```python
from build123d import *

# Parameters (mm, degrees)
SKETCH2_W               = 85
SKETCH2_H               = 115
BOSS_EXTRUDE1_DEPTH     = 15
SKETCH3_W               = 15
SKETCH3_H               = 4.5
CUT_EXTRUDE1_DEPTH      = 144.788038445
MIRROR2_COPY_1_SKETCH_W = 15
MIRROR2_COPY_1_SKETCH_H = 4.5
MIRROR2_COPY_1_DEPTH    = 144.788038445
SKETCH4_W               = 55
SKETCH4_H               = 115
BOSS_EXTRUDE2_DEPTH     = 2
SKETCH6_W               = 55
SKETCH6_H               = 115
CUT_EXTRUDE2_DEPTH      = 4.5
SKETCH5_W               = 85
SKETCH5_H               = 115
BOSS_EXTRUDE3_DEPTH     = 4


with BuildPart() as part:
    # Sketch2 → Boss-Extrude1 (new body)
    with BuildSketch(Plane.XY):
        with Locations((42.5, 57.5)):
            Rectangle(SKETCH2_W, SKETCH2_H)
    extrude(amount=BOSS_EXTRUDE1_DEPTH)

    # Sketch3 → Cut-Extrude1 (cut, through all)
    with BuildSketch(Plane(origin=(0, 115, 0), x_dir=(1, 0, 0), z_dir=(0, 1, 0))):
        with Locations((7.5, -12.75)):
            Rectangle(SKETCH3_W, SKETCH3_H)
    cut_extrude1 = extrude(amount=-CUT_EXTRUDE1_DEPTH, mode=Mode.SUBTRACT)

    # Mirror1: Cut-Extrude1 across plane
    add(cut_extrude1.mirror(Plane.XY.offset(7.5)), mode=Mode.SUBTRACT)

    # Mirror2: Cut-Extrude1 across plane
    add(cut_extrude1.mirror(Plane.ZY.offset(-42.5)), mode=Mode.SUBTRACT)

    # Mirror2 copy 1 sketch → Mirror2 copy 1 (cut, through all)
    with BuildSketch(Plane(origin=(85, 115, 15), x_dir=(-1, 0, 0), z_dir=(0, 1, 0))):
        with Locations((7.5, -12.75)):
            Rectangle(MIRROR2_COPY_1_SKETCH_W, MIRROR2_COPY_1_SKETCH_H)
    extrude(amount=-MIRROR2_COPY_1_DEPTH, mode=Mode.SUBTRACT)

    # Sketch4 → Boss-Extrude2 (add)
    with BuildSketch(Plane.XY.offset(15)):
        with Locations((42.5, 57.5)):
            Rectangle(SKETCH4_W, SKETCH4_H)
    extrude(amount=BOSS_EXTRUDE2_DEPTH)

    # Sketch6 → Cut-Extrude2 (cut)
    with BuildSketch(Plane(origin=(0, 0, 0), x_dir=(-1, 0, 0), z_dir=(0, 0, -1))):
        with Locations((-42.5, 57.5)):
            Rectangle(SKETCH6_W, SKETCH6_H)
    extrude(amount=-CUT_EXTRUDE2_DEPTH, mode=Mode.SUBTRACT)

    # Sketch5 → Boss-Extrude3 (add)
    with BuildSketch(Plane.XY.offset(17)):
        with Locations((42.5, 57.5)):
            Rectangle(SKETCH5_W, SKETCH5_H)
    extrude(amount=BOSS_EXTRUDE3_DEPTH)


solid = part.part
```
Input: part model. Units: mm. Frame: model coordinates. A direction names the side the tool comes from. Round coordinates to 2 decimals unless told otherwise and drop trailing zeros. Loops run counter-clockwise (first coordinate to the right, second up) from the corner with the lowest first, then second, coordinate; pieces in that order, holes last. Notation, with made-up numbers: M 88,11.5 L 127,11.5 A10 ccw 127,15.5 Z; hole C 39,8 d8. An arc over 180 degrees is marked long. Answer in a Markdown table with one row per item. Add a question column.
1. Contact query for a flat-ended pin moving along its axis: pin 1 (2 mm diameter, centred on y = 30.5, z = 15, fed in from -X). Output: stop coordinate, or through.
2. Section C-C (z = 15.5). Output: boundary loops of the cut face in (x, y), and give its area (4 significant figures).
3. Section A-A (x = 6). Output: boundary loops of the cut face in (y, z).
4. Set-up query: faces 1 (the face through (15, 57, 14)), 2 (the face through (77, 58, 17)), 3 (the face through (85, 57, 7)). Return all of +Z, -Z, +X, -X, +Y, -Y with unobstructed straight access to the full face (end or side cutting, diameter ignored); none if empty.
5. Section B-B (y = 75). Output: boundary loops of the cut face in (x, z), and give its area (3 significant figures).
6. Mould query, pull axis Z, two halves, no side actions, for faces 4 (the face through (7, 58, 10.5)), 5 (the face through (42, 115, 13)), 6 (the face through (42, 58, 4.5)). Classes: released by +Z, released by -Z, zero draft, split by the parting line, or undercut.
7. Ray query, probe 1 along Z at (x, y) = (7, 26.5); probe 2 along X at (y, z) = (27.5, 16.75). Return the intervals inside material, ascending.
Values follow:
| question | item | result |
|---|---|---|
| 1 | pin 1 | x = 15 |
| 2 | outline | M 15,0 L 70,0 L 70,115 L 15,115 Z |
| 2 | area | 6,325 mm^2 |
| 3 | outline | M 0,4.5 L 115,4.5 L 115,10.5 L 0,10.5 Z; M 0,17 L 115,17 L 115,21 L 0,21 Z |
| 4 | face 1 | -X, +Y, -Y |
| 4 | face 2 | +X, +Y, -Y |
| 4 | face 3 | +Z, -Z, +X, +Y, -Y |
| 5 | outline | M 0,4.5 L 85,4.5 L 85,10.5 L 70,10.5 L 70,17 L 85,17 L 85,21 L 0,21 L 0,17 L 15,17 L 15,10.5 L 0,10.5 Z |
| 5 | area | 1,210 mm^2 |
| 6 | face 4 | undercut |
| 6 | face 5 | zero draft |
| 6 | face 6 | released by -Z |
| 7 | probe 1 | 4.5 to 10.5, 17 to 21 |
| 7 | probe 2 | 15 to 70 |
